The listing builds one solid part. Answer for the finished solid, in the listing's coordinates (mm). A direction names the side the tool comes from. Coordinates: 2 decimals unless noted, no trailing zeros. Loops run counter-clockwise (first coordinate to the right, second up) from the corner with the lowest first, then second, coordinate; pieces in that order, holes last. Notation, with made-up numbers: (69, -16.75) - (92, -16.75) arc R19 cw to (92, 12.25) - close; hole circle Ø9 at (77.25, 88.25). An arc over 180 degrees is marked (long way). One line per question, with ' | ' between items.
Autodesk Fusion 360 part; units mm, degrees
sketch "Boceto1" plane through (0, 0, 0) normal (0, 1, 0) x (1, 0, 0)
  line L0 (16.7, -13.25) -> (-16.7, -13.25)
  line L1 (-16.7, -13.25) -> (-16.7, 13.25)
  line L2 (-16.7, 13.25) -> (16.7, 13.25)
  line L3 (16.7, 13.25) -> (16.7, -13.25)
  line L4 (16.7, -13.25) -> (-16.7, 13.25) construction
  line L5 (-16.7, -13.25) -> (16.7, 13.25) construction
  line L6 (-14.4, 8.65) -> (12.2, 8.65)
  line L7 (12.2, 8.65) -> (12.2, -6.65)
  line L8 (12.2, -6.65) -> (-14.4, -6.65)
  line L9 (-14.4, -6.65) -> (-14.4, 8.65)
  line L10 (-6.4, 8.65) -> (-6.4, -6.65)
  circle A0 centre (-14.85, 11.4) radius 1.35
  circle A1 centre (14.85, 11.4) radius 1.35
  circle A2 centre (14.85, -11.4) radius 1.35
  circle A3 centre (-14.85, -11.4) radius 1.35
  line L11 (14.4, 8.25) -> (16.7, 8.25)
  line L12 (16.7, 8.25) -> (16.7, 0.95)
  line L13 (16.7, 0.95) -> (14.4, 0.95)
  line L14 (14.4, 0.95) -> (14.4, 8.25)
  dimension "d1" = 33.4
  dimension "d2" = 26.5
  dimension "d3" = 26.6
  dimension "d4" = 15.3
  dimension "d5" = 4.6
  dimension "d6" = 4.5
  dimension "d8" = 8
  dimension "d16" = 2.7
  dimension "d17" = 1.85
  dimension "d18" = 1.85
  dimension "d19" = 1.85
  dimension "d20" = 1.85
  dimension "d21" = 5
  dimension "d22" = 2.3
  dimension "d23" = 7.3
extrude "Extruir1" add sketch "Boceto1" along normal blind 3.6 contours L0 L1 L2 L3 L11 L13 L14 | L3 L11 L12 L13 L14 | L6 L8 L9 L10 | L6 L7 L8 L10
extrude "Extruir2" add sketch "Boceto1" along normal blind 17.9 contours L6 L7 L8 L10
extrude "Extruir3" add sketch "Boceto1" along normal blind 13 contours L6 L8 L9 L10
chamfer "Chaflán1" distance 2 angle 45 1 edges at (-14.4, 13, -1)
extrude "Extruir4" add sketch "Boceto1" along normal blind 6 contours L3 L11 L12 L13 L14
sketch "Boceto2" plane through (16.7, 0, 0) normal (1, 0, 0) x (0, 0, -1)
  line L0 (0.95, 3.6) -> (-13.25, 3.6)
  line L1 (-13.25, 3.6) -> (-13.25, 0)
  line L2 (-13.25, 0) -> (13.25, 0)
  line L3 (13.25, 0) -> (13.25, 3.6)
  line L4 (13.25, 3.6) -> (8.25, 3.6)
  line L5 (8.25, 3.6) -> (8.25, 6)
  line L6 (8.25, 6) -> (0.95, 6)
  line L7 (0.95, 6) -> (0.95, 3.6)
  line L8 (1.85, 6) -> (7.35, 6)
  line L9 (7.35, 6) -> (7.35, 5.4)
  line L10 (7.35, 5.4) -> (1.85, 5.4)
  line L11 (1.85, 5.4) -> (1.85, 6)
  point P0 (4.6, 6)
  point P1 (4.6, 6)
  dimension "d26" = 0.6
  dimension "d27" = 5.5
extrude "Extruir5" add sketch "Boceto2" along normal blind 6.8 contours L6 L8 L9 L10 L11
equation "d9 = 1.2 mm + 2.4 mm"
equation "d11 = 16.7 mm + 1.2 mm"
equation "d17 = 0.5 mm + ( ( 2.7 / 2 ) * 1 mm )"
equation "d18 = 0.5 mm + ( ( 2.7 / 2 ) * 1 mm )"
equation "d19 = 0.5 mm + ( ( 2.7 / 2 ) * 1 mm )"
equation "d20 = 0.5 mm + ( ( 2.7 / 2 ) * 1 mm )"
Item 1: Find section D-D, the plane x = -4.5. Write down the section's boundary in (y, z), plus the area to 3 significant figures.
Taken from the geometry:
outline: (0, -13.25) - (3.6, -13.25) - (3.6, -8.65) - (17.9, -8.65) - (17.9, 6.65) - (3.6, 6.65) - (3.6, 13.25) - (0, 13.25) - close | area: 314 mm2
Item 2: Each of these flat-tipped pins is pushed along its axis until it touches: pin 1 Ø3 at (x, z) = (-14.85, 11.4) entering from +Y; pin 2 Ø3 at (x, z) = (-8, 2.5) entering from +Y; pin 3 Ø3 at (y, z) = (2.5, -3) entering from +X; pin 4 Ø2 at (x, z) = (-14.85, -11.4) entering from +Y. Where does it stop, or does it pass through?
Taken from the geometry:
pin 1: stops at y = 3.6 | pin 2: stops at y = 13 | pin 3: stops at x = 16.7 | pin 4: passes through
Item 3: Find section A-A, the plane z = 11.4. Write down the section's boundary in (x, y), plus the area to 3 significant figures.
Taken from the geometry:
outline: (-16.7, 0) - (-16.2, 0) - (-16.2, 3.6) - (-16.7, 3.6) - close; (-13.5, 0) - (13.5, 0) - (13.5, 3.6) - (-13.5, 3.6) - close; (16.2, 0) - (16.7, 0) - (16.7, 3.6) - (16.2, 3.6) - close | area: 101 mm2
Item 4: The mould has two halves that part along X. Classify faces 1 (the face through (14.56, 1.77, 10.08)), 2 (the face through (-13.4, 12, -1.1)), 3 (the face through (0, 2, 13.25)): pulls with the +X half, pulls with the -X half, needs draft (parallel to the pull), parting line crosses it, or undercut.
Taken from the geometry:
face 1: undercut | face 2: pulls with the -X half | face 3: needs draft
Item 5: Which of the six approach directions +Z, -Z, +X, -X, +Y, -Y give full straight-line access (tool end or side, diameter ignored) to faces 4 (the face through (14.4, 5, -5)), 5 (the face through (-14.4, 7, -1)), 6 (the face through (-1, 11, 6.65))?
Taken from the geometry:
face 4: +Z, -Z, +Y | face 5: +Z, -Z, -X, +Y | face 6: +Z, +X, -X, +Y
Item 6: Find section C-C, the plane z = -6. Write down the section's boundary in (x, y).
Taken from the geometry:
outline: (-16.7, 0) - (16.7, 0) - (16.7, 5.4) - (23.5, 5.4) - (23.5, 6) - (14.4, 6) - (14.4, 3.6) - (12.2, 3.6) - (12.2, 17.9) - (-6.4, 17.9) - (-6.4, 13) - (-12.4, 13) - (-14.4, 11) - (-14.4, 3.6) - (-16.7, 3.6) - close
Item 7: Find section B-B, the plane x = 14.85. Write down the section's boundary in (y, z), plus the area to 3 significant figures.
Taken from the geometry:
outline: (0, -13.25) - (3.6, -13.25) - (3.6, -12.75) - (0, -12.75) - close; (0, -10.05) - (3.6, -10.05) - (3.6, -8.25) - (6, -8.25) - (6, -0.95) - (3.6, -0.95) - (3.6, 10.05) - (0, 10.05) - close; (0, 12.75) - (3.6, 12.75) - (3.6, 13.25) - (0, 13.25) - close | area: 93.5 mm2
Item 8: Find the intervals of material crossed by line 1 (Z direction, x = -14.85, y = 0.9); line 2 (X direction, y = 1.3, z = 11.4); line 3 (Y direction, x = -9, z = 8.75), in increasing order. Write a range as [from, to].
Taken from the geometry:
line 1: z = [-13.25, -12.75], [-10.05, 10.05], [12.75, 13.25] | line 2: x = [-16.7, -16.2], [-13.5, 13.5], [16.2, 16.7] | line 3: y = [0, 3.6]
